Study the drawing (mm; zero at the part's minimum x, y, z) and answer. A direction names the side the tool comes from. Coordinates: 2 decimals unless noted, no trailing zeros. Order: outer loops, then holes, each group sorted by start corner. A loop starts at its lowest first (then second) coordinate and runs counter-clockwise, first axis right, second up.
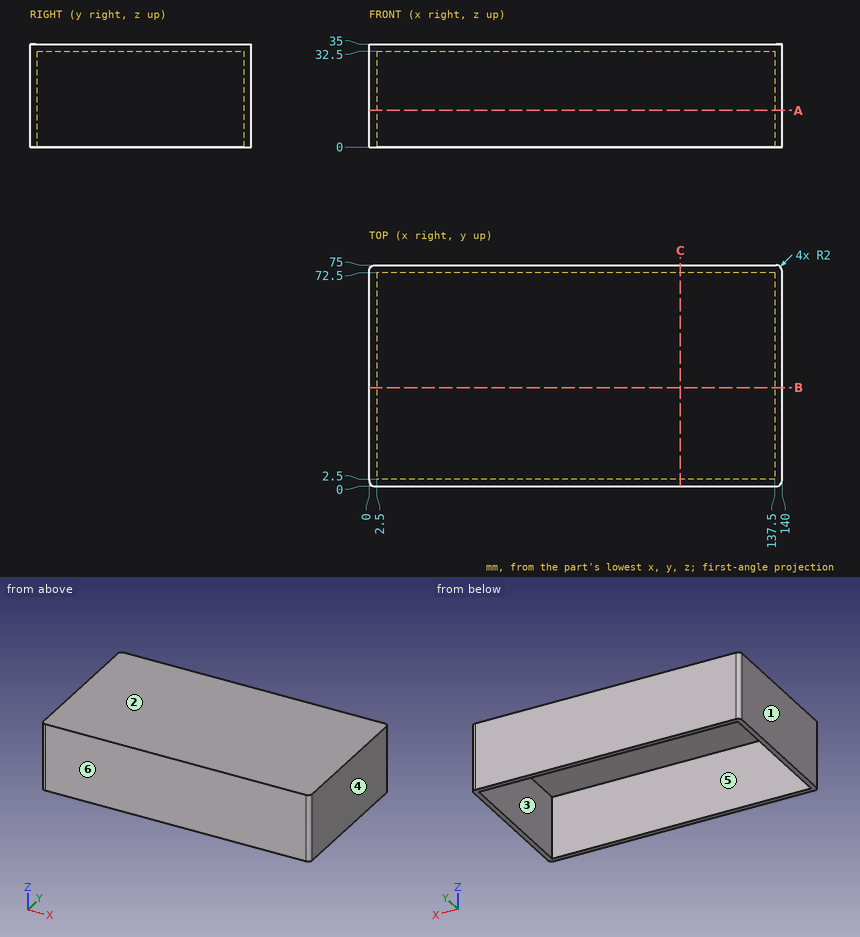
1) A cutting plane is placed at A-A, the plane z = 12.5. Determine the outline of the cut face in (x, y).
A:
outline: (0, 2) arc R2 ccw to (2, 0) - (138, 0) arc R2 ccw to (140, 2) - (140, 73) arc R2 ccw to (138, 75) - (2, 75) arc R2 ccw to (0, 73) - close; hole (2.5, 2.5) - (137.5, 2.5) - (137.5, 72.5) - (2.5, 72.5) - close
2) Straight lines are drawn through the part: line 1 (X direction, y = 32, z = 22.5); line 2 (Y direction, x = 55, z = 13.5); line 3 (Z direction, x = 98.5, y = 45). For each, find the intervals that lie inside material, in ascending order.
A:
line 1: x = 0 to 2.5, 137.5 to 140
line 2: y = 0 to 2.5, 72.5 to 75
line 3: z = 32.5 to 35
3) A cutting plane is placed at B-B, the plane y = 33.5. Determine the outline of the cut face in (x, z).
A:
outline: (0, 0) - (2.5, 0) - (2.5, 32.5) - (137.5, 32.5) - (137.5, 0) - (140, 0) - (140, 35) - (0, 35) - close
4) Determine the mould class of the marked faces 1, 2, 3 and 4 for opening direction X: pulls with the +X half, pulls with the -X half, needs draft (parallel to the pull), parting line crosses it, or undercut.
A:
face 1: pulls with the -X half
face 2: needs draft
face 3: undercut
face 4: pulls with the +X half
5) A cutting plane is placed at C-C, the plane x = 105.5. Determine the outline of the cut face in (y, z).
A:
outline: (0, 0) - (2.5, 0) - (2.5, 32.5) - (72.5, 32.5) - (72.5, 0) - (75, 0) - (75, 35) - (0, 35) - close
6) A flat-ended cylindrical pin translates along its axis: pin 1 Ø6 at (x, y) = (110, 59) entering from -Z. Find the tip coordinate at first contact, or state that the pin passes through.
A:
pin 1: stops at z = 32.5
7) Which of the six approach directions +Z, -Z, +X, -X, +Y, -Y give full straight-line access (tool end or side, diameter ignored) to the marked faces 5 and 6?
A:
face 5: -Z
face 6: +Z, -Z, +X, -X, -Y
